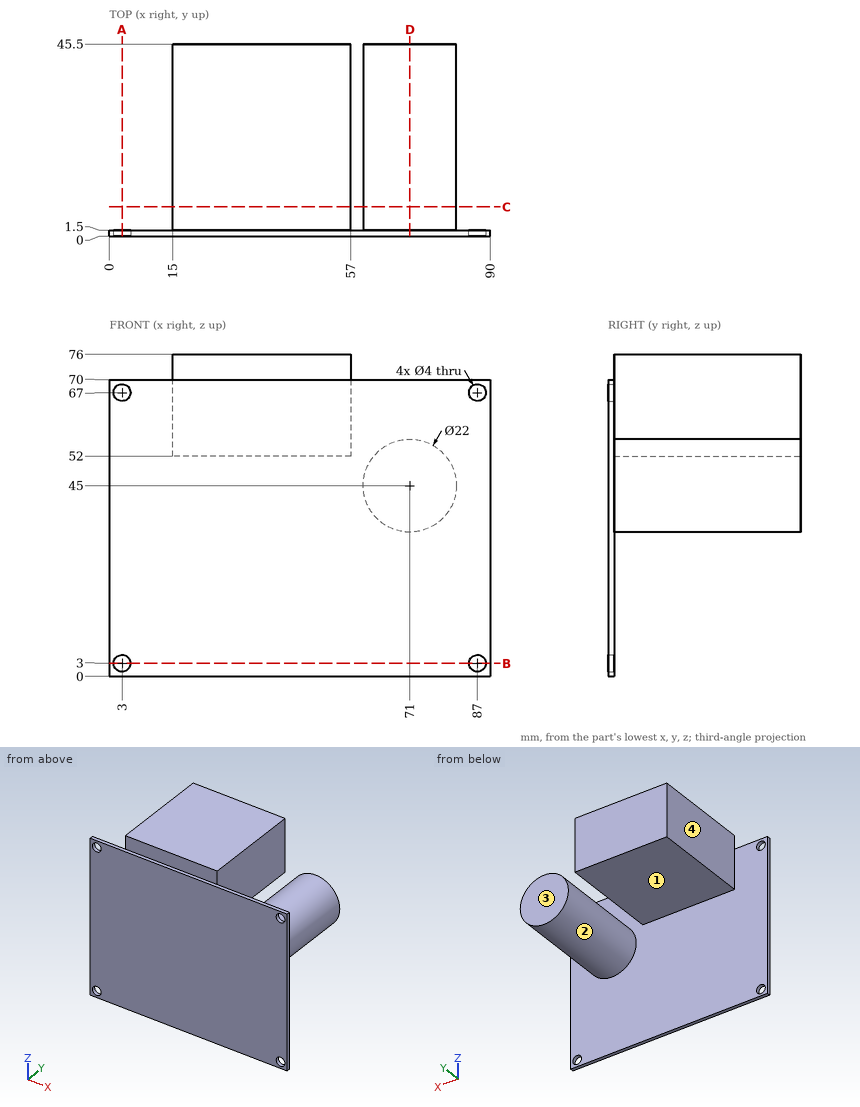
Answer from the drawing. Dimensions are ordinates in mm from the lowest x, y and z of the part. A direction names the side the tool comes from. Give positions to 0.01 mm unless a question says otherwise; leave off trailing zeros. Order: outer loops, then holes, each group sorted by start corner. A loop starts at its lowest first (then second) coordinate and runs counter-clockwise, first axis right, second up.
(1) Find section D-D (x = 71). Give the vertices of the cut face in (y, z).
(2) Find section A-A (x = 3). Give the vertices of the cut face in (y, z).
(3) For the marked faces 1, 2, 3 and 4, determine the directions among +Z, -Z, +X, -X, +Y, -Y from which every point of the face is accessible in a straight line to the end or side of a thin tool.
(4) Find section B-B (z = 3). Give the vertices of the cut face in (x, y), plus the area to 3 significant figures.
(5) Straight lines are drawn through the part: L1, parallel to Z at x = 3, y = 1; L2, parallel to X at y = 0.75, z = 3; L3, parallel to Y at x = 35, z = 33.5. For each, find the intervals that lie inside material, in ascending order.
(6) Given pin 1 (8 mm diameter, centred on x = 49, y = 35, fed in from -Z); pin 2 (2 mm diameter, centred on x = 73.5, y = 22, fed in from -Z); pin 3 (19 mm diameter, centred on y = 18, z = 66.5, fed in from -X), each flat-ended and moving along its own axis, determine where each tip first touches the part or whether it passes through.
(7) Find section C-C (y = 7). Give the vertices of the cut face in (x, z), plus the area to 3 significant figures.
Result sheet:
1. outline: (0, 0) - (1.5, 0) - (1.5, 34) - (45.5, 34) - (45.5, 56) - (1.5, 56) - (1.5, 70) - (0, 70) - close
2. outline: (0, 0) - (1.5, 0) - (1.5, 1) - (0, 1) - close; (0, 5) - (1.5, 5) - (1.5, 65) - (0, 65) - close; (0, 69) - (1.5, 69) - (1.5, 70) - (0, 70) - close
3. face 1: -Z, -X, +Y
3. face 2: +Y
3. face 3: +Z, -Z, +X, -X, +Y
3. face 4: +Z, -Z, -X, +Y
4. outline: (0, 0) - (1, 0) - (1, 1.5) - (0, 1.5) - close; (5, 0) - (85, 0) - (85, 1.5) - (5, 1.5) - close; (89, 0) - (90, 0) - (90, 1.5) - (89, 1.5) - close
4. area: 123 mm2
5. L1: z = 0 to 1, 5 to 65, 69 to 70
5. L2: x = 0 to 1, 5 to 85, 89 to 90
5. L3: y = 0 to 1.5
6. pin 1: stops at z = 52
6. pin 2: stops at z = 34.1
6. pin 3: stops at x = 15
7. outline: (15, 52) - (57, 52) - (57, 76) - (15, 76) - close; circle Ø22 at (71, 45)
7. area: 1,390 mm2
